```python
from build123d import *

# Parameters (mm, degrees)
SKETCH3_W                 = 120
SKETCH3_H                 = 200
SKETCH3_R                 = 1.38
BOSS_EXTRUDE1_DEPTH       = 2
BOSS_EXTRUDE2_DEPTH       = 120
SKETCH5_R                 = 1.38
CUT_EXTRUDE1_DEPTH        = 7.16
SKETCH7_R                 = 4.998737833
SKETCH7_R_2               = 7.554686589
SKETCH7_R_3               = 5.693928521
SKETCH7_R_4               = 3.338756268
SKETCH7_R_5               = 5.843083046
SKETCH7_R_6               = 5.380127949
SKETCH7_R_7               = 4.59382227
SKETCH7_R_8               = 2.636652122
SKETCH7_R_9               = 5.065111982
CUT_EXTRUDE2_DEPTH        = 7.16
MIRROR2_COPY_1_SKETCH_R   = 4.998737833
MIRROR2_COPY_1_SKETCH_R_2 = 7.554686589
MIRROR2_COPY_1_SKETCH_R_3 = 5.693928521
MIRROR2_COPY_1_SKETCH_R_4 = 3.338756268
MIRROR2_COPY_1_SKETCH_R_5 = 5.843083046
MIRROR2_COPY_1_SKETCH_R_6 = 5.380127949
MIRROR2_COPY_1_SKETCH_R_7 = 4.59382227
MIRROR2_COPY_1_SKETCH_R_8 = 2.636652122
MIRROR2_COPY_1_SKETCH_R_9 = 5.065111982
MIRROR2_COPY_1_DEPTH      = 7.16
SKETCH8_R                 = 2.55
CUT_EXTRUDE3_DEPTH        = 7.16


with BuildPart() as part:
    # Sketch3 → Boss-Extrude1 (new body)
    with BuildSketch(Plane(origin=(0, 0, 0), x_dir=(1, 0, 0), z_dir=(0, 1, 0))):
        with Locations((1e-09, 0)):
            Rectangle(SKETCH3_W, SKETCH3_H)
        with Locations((-43, 29)):
            Circle(SKETCH3_R, mode=Mode.SUBTRACT)
        with Locations((43, 29)):
            Circle(SKETCH3_R, mode=Mode.SUBTRACT)
        with Locations((43, -29)):
            Circle(SKETCH3_R, mode=Mode.SUBTRACT)
        with Locations((-43, -29)):
            Circle(SKETCH3_R, mode=Mode.SUBTRACT)
    extrude(amount=BOSS_EXTRUDE1_DEPTH)

    # Sketch4 → Boss-Extrude2 (add)
    with BuildSketch(Plane.ZY.offset(59.999999999)):
        Polygon((-89.35, 0), (-91.75177712, -4.16), (-79.34822288, -4.16), (-81.75, 0), align=None)
        Polygon((81.75, 0), (79.34822288, -4.16), (91.75177712, -4.16), (89.35, 0), align=None)
    extrude(amount=-BOSS_EXTRUDE2_DEPTH)

    # Sketch5 → Cut-Extrude1 (cut, through all)
    with BuildSketch(Plane(origin=(0, 2, 0), x_dir=(1, 0, 0), z_dir=(0, 1, 0))):
        with Locations((-10, -86)):
            Circle(SKETCH5_R)
        with Locations((10, -86)):
            Circle(SKETCH5_R)
        with Locations((-45.999999999, 10)):
            Circle(SKETCH5_R)
        with Locations((-45.999999999, -10)):
            Circle(SKETCH5_R)
        with Locations((-25.999999999, 10)):
            Circle(SKETCH5_R)
        with Locations((-25.999999999, -10)):
            Circle(SKETCH5_R)
        with Locations((26.000000001, 10)):
            Circle(SKETCH5_R)
        with Locations((26.000000001, -10)):
            Circle(SKETCH5_R)
        with Locations((46.000000001, 10)):
            Circle(SKETCH5_R)
        with Locations((46.000000001, -10)):
            Circle(SKETCH5_R)
        with Locations((-10, -66)):
            Circle(SKETCH5_R)
        with Locations((10, -66)):
            Circle(SKETCH5_R)
        with Locations((-10, 86)):
            Circle(SKETCH5_R)
        with Locations((10, 86)):
            Circle(SKETCH5_R)
        with Locations((-10, 66)):
            Circle(SKETCH5_R)
        with Locations((10, 66)):
            Circle(SKETCH5_R)
    extrude(amount=-CUT_EXTRUDE1_DEPTH, mode=Mode.SUBTRACT)

    # Sketch7 → Cut-Extrude2 (cut, through all)
    with BuildSketch(Plane(origin=(0, 2, 0), x_dir=(1, 0, 0), z_dir=(0, 1, 0))):
        with Locations((-22.521130628, -38.521841888)):
            Circle(SKETCH7_R)
        with Locations((-35.576157364, -49.846684357)):
            Circle(SKETCH7_R_2)
        with Locations((-15.770265305, -53.307052889)):
            Circle(SKETCH7_R_3)
        with Locations((-38.779208604, -66.765189198)):
            Circle(SKETCH7_R_4)
        with Locations((-22.835709586, -69.350579721)):
            Circle(SKETCH7_R_5)
        with Locations((-15.770265305, -23.019185403)):
            Circle(SKETCH7_R_2)
        with Locations((-8.050498584, -38.521841888)):
            Circle(SKETCH7_R_6)
        with Locations((-11.079773886, -7.545708078)):
            Circle(SKETCH7_R_7)
        with Locations((-34.317841534, -35.218762834)):
            Circle(SKETCH7_R_8)
        with Locations((-33.216815183, -21.062709748)):
            Circle(SKETCH7_R)
        with Locations((-47.058289312, -39.150999803)):
            Circle(SKETCH7_R_9)
        with Locations((-47.058289312, -53.307052889)):
            Circle(SKETCH7_R_8)
    cut_extrude2 = extrude(amount=-CUT_EXTRUDE2_DEPTH, mode=Mode.SUBTRACT)

    # Mirror1: Cut-Extrude2 across plane
    add(cut_extrude2.mirror(Plane.XY), mode=Mode.SUBTRACT)

    # Mirror2: Cut-Extrude2 across plane
    add(cut_extrude2.mirror(Plane(origin=(0, 0, 0), x_dir=(0, 0, 1), z_dir=(1, 0, 0))), mode=Mode.SUBTRACT)

    # Mirror2 copy 1 sketch → Mirror2 copy 1 (cut, through all)
    with BuildSketch(Plane(origin=(0, 2, 0), x_dir=(-1, 0, 0), z_dir=(0, 1, 0))):
        with Locations((-22.521130628, -38.521841888)):
            Circle(MIRROR2_COPY_1_SKETCH_R)
        with Locations((-35.576157364, -49.846684357)):
            Circle(MIRROR2_COPY_1_SKETCH_R_2)
        with Locations((-15.770265305, -53.307052889)):
            Circle(MIRROR2_COPY_1_SKETCH_R_3)
        with Locations((-38.779208604, -66.765189198)):
            Circle(MIRROR2_COPY_1_SKETCH_R_4)
        with Locations((-22.835709586, -69.350579721)):
            Circle(MIRROR2_COPY_1_SKETCH_R_5)
        with Locations((-15.770265305, -23.019185403)):
            Circle(MIRROR2_COPY_1_SKETCH_R_2)
        with Locations((-8.050498584, -38.521841888)):
            Circle(MIRROR2_COPY_1_SKETCH_R_6)
        with Locations((-11.079773886, -7.545708078)):
            Circle(MIRROR2_COPY_1_SKETCH_R_7)
        with Locations((-34.317841534, -35.218762834)):
            Circle(MIRROR2_COPY_1_SKETCH_R_8)
        with Locations((-33.216815183, -21.062709748)):
            Circle(MIRROR2_COPY_1_SKETCH_R)
        with Locations((-47.058289312, -39.150999803)):
            Circle(MIRROR2_COPY_1_SKETCH_R_9)
        with Locations((-47.058289312, -53.307052889)):
            Circle(MIRROR2_COPY_1_SKETCH_R_8)
    extrude(amount=-MIRROR2_COPY_1_DEPTH, mode=Mode.SUBTRACT)

    # Sketch8 → Cut-Extrude3 (cut, through all)
    with BuildSketch(Plane.XZ.offset(4.16)):
        with Locations((1e-09, 85.55)):
            Circle(SKETCH8_R)
    cut_extrude3 = extrude(amount=-CUT_EXTRUDE3_DEPTH, mode=Mode.SUBTRACT)

    # Mirror3: Cut-Extrude3 across plane
    add(cut_extrude3.mirror(Plane.XY), mode=Mode.SUBTRACT)


solid = part.part
```
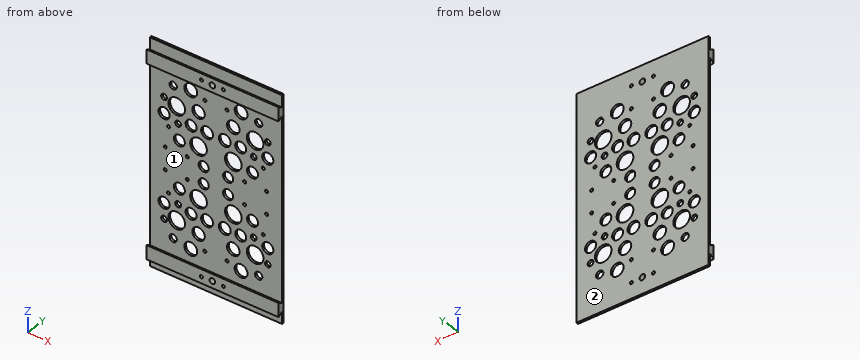
For this review, take the finished solid that the model builds, in its own axes (mm). Face numbers are marked on the shaded views. Coordinates: 2 decimals unless noted, no trailing zeros. Order: outer loops, then holes, each group sorted by start corner. A loop starts at its lowest first (then second) coordinate and runs counter-clockwise, first axis right, second up. Notation, with made-up numbers: (53.5, -10.5) - (109.5, -10.5) arc R30 cw to (109.5, 17.5) - close; hole circle Ø9 at (-25, -24.75). An arc over 180 degrees is marked (long way). Answer as a JSON object with one key per item and string values. Group by question number.
1. For probe 1 along Z at (x, y) = (-41.5, 0.5); probe 2 along Z at (x, y) = (0, -1.75); probe 3 along Y at (x, z) = (-8, 48.5), list the stretches that pass through material, from the lowest coordinate up.
2. We need section A-A on x = 0. State the section outline as (y, z) points, then the cut area to 3 significant figures.
3. The part is to be moulded in two halves that separate along Z. For the marked faces 1 and 2, say which applies: pulls with the +Z half, pulls with the -Z half, needs draft (parallel to the pull), parting line crosses it, or undercut.
4. Clearance check with flat-ended pins moving along their axes: P1, Ø6, axis at x = 21, z = 33.5, coming from the -Y side; P2, Ø8.5, axis at x = 47.06, z = 53.31, coming from the +Y side; P3, Ø4.5, axis at x = -34.32, z = 35.22, coming from the -Y side. State where each tip first meets the part, or that it passes through.
5. We need section B-B on y = -2.25. State the section outline as (x, z) points.
Final values:
{
 "1": {"probe 1": "-100 to -68.7, -64.83 to -54.54, -45.16 to 45.16, 54.54 to 64.83, 68.7 to 100", "probe 2": "-90.36 to -88.1, -83 to -80.74, 80.74 to 83, 88.1 to 90.36", "probe 3": "0 to 2"},
 "2": {"outline": "(-4.16, -91.75) - (0, -89.35) - (0, -100) - (2, -100) - (2, -88.1) - (-4.16, -88.1) - close; (-4.16, -83) - (2, -83) - (2, 83) - (-4.16, 83) - (-4.16, 79.35) - (0, 81.75) - (0, -81.75) - (-4.16, -79.35) - close; (-4.16, 88.1) - (2, 88.1) - (2, 100) - (0, 100) - (0, 89.35) - (-4.16, 91.75) - close", "area": "420 mm²"},
 "3": {"face 1": "undercut", "face 2": "needs draft"},
 "4": {"P1": "y = 0", "P2": "y = 2", "P3": "through"},
 "5": {"outline": "(-60, -90.65) - (60, -90.65) - (60, -80.45) - (-60, -80.45) - close; (-60, 80.45) - (60, 80.45) - (60, 90.65) - (-60, 90.65) - close; hole circle Ø2.76 at (-10, -86); hole circle Ø2.76 at (-10, 86); hole circle Ø5.1 at (0, -85.55); hole circle Ø5.1 at (0, 85.55); hole circle Ø2.76 at (10, -86); hole circle Ø2.76 at (10, 86)"}
}
